from build123d import *

# Parameters (mm, degrees)
SKETCH_1_R          = 6.15
EXTRUDE_1_DEPTH     = 0.2
SKETCH_2_R          = 2.8
EXTRUDE_2_DEPTH     = 0.9
SKETCH_3_R          = 6.15
EXTRUDE_3_DEPTH     = 1.1
EXTRUDE_START       = -0.6
SKETCH_4_R          = 6.15
EXTRUDE_4_DEPTH     = 0.6
CUT_EXTRUDE_START   = -0.2
SKETCH_6_R          = 3.55
SKETCH_6_R_2        = 2.8
CUT_EXTRUDE_2_DEPTH = 0.2
EXTRUDE_START_2     = 7
SKETCH_7_R          = 6.15
SKETCH_7_R_2        = 4.75
EXTRUDE_5_DEPTH     = 7
CHAMFER_4_SIZE      = 2.5
CHAMFER_5_SIZE      = 0.4
CHAMFER_6_SIZE      = 0.4
CHAMFER_7_SIZE      = 1
CHAMFER_8_SIZE      = 0.3


with BuildPart() as part:
    # Sketch 1 → Extrude 1 (new body)
    with BuildSketch(Plane.XY):
        Circle(SKETCH_1_R)
        with BuildLine():
            Line((-0.6, 5.25), (0, 5.85))
            Line((0, 5.85), (0.6, 5.25))
            Line((0.6, 5.25), (0.6, 1.670516387))
            ThreePointArc((0.6, 1.670516387), (0.8875, 1.537195092), (1.146709629, 1.354873436))
            Line((1.146709629, 1.354873436), (4.24663337, 3.144615242))
            Line((4.24663337, 3.144615242), (5.066248612, 2.925))
            Line((5.066248612, 2.925), (4.84663337, 2.105384758))
            Line((4.84663337, 2.105384758), (1.746709629, 0.315642951))
            ThreePointArc((1.746709629, 0.315642951), (1.76791326, 0.158454108), (1.775, 0))
            ThreePointArc((1.775, 0), (1.76791326, -0.158454108), (1.746709629, -0.315642951))
            Line((1.746709629, -0.315642951), (4.84663337, -2.105384758))
            Line((4.84663337, -2.105384758), (5.066248612, -2.925))
            Line((5.066248612, -2.925), (4.24663337, -3.144615242))
            Line((4.24663337, -3.144615242), (1.146709629, -1.354873436))
            ThreePointArc((1.146709629, -1.354873436), (0.8875, -1.537195092), (0.6, -1.670516387))
            Line((0.6, -1.670516387), (0.6, -5.25))
            Line((0.6, -5.25), (0, -5.85))
            Line((0, -5.85), (-0.6, -5.25))
            Line((-0.6, -5.25), (-0.6, -1.670516387))
            ThreePointArc((-0.6, -1.670516387), (-0.8875, -1.537195092), (-1.146709629, -1.354873436))
            Line((-1.146709629, -1.354873436), (-4.24663337, -3.144615242))
            Line((-4.24663337, -3.144615242), (-5.066248612, -2.925))
            Line((-5.066248612, -2.925), (-4.84663337, -2.105384758))
            Line((-4.84663337, -2.105384758), (-1.746709629, -0.315642951))
            ThreePointArc((-1.746709629, -0.315642951), (-1.775, 0), (-1.746709629, 0.315642951))
            Line((-1.746709629, 0.315642951), (-4.84663337, 2.105384758))
            Line((-4.84663337, 2.105384758), (-5.066248612, 2.925))
            Line((-5.066248612, 2.925), (-4.24663337, 3.144615242))
            Line((-4.24663337, 3.144615242), (-1.146709629, 1.354873436))
            ThreePointArc((-1.146709629, 1.354873436), (-0.8875, 1.537195092), (-0.6, 1.670516387))
            Line((-0.6, 1.670516387), (-0.6, 5.25))
        make_face(mode=Mode.SUBTRACT)
    extrude(amount=EXTRUDE_1_DEPTH)

    # Sketch 3 → Extrude 3 (add)
    with BuildSketch(Plane.XY.offset(0.2)):
        Circle(SKETCH_3_R)
        with BuildLine():
            Line((-4.933776406, -2.430606997), (-5.066248612, -2.925))
            Line((-5.066248612, -2.925), (-4.571855609, -3.057472206))
            ThreePointArc((-4.571855609, -3.057472206), (-2.75, -4.763139721), (-0.361920797, -5.488079203))
            Line((-0.361920797, -5.488079203), (0, -5.85))
            Line((0, -5.85), (0.361920797, -5.488079203))
            ThreePointArc((0.361920797, -5.488079203), (2.75, -4.763139721), (4.571855609, -3.057472206))
            Line((4.571855609, -3.057472206), (5.066248612, -2.925))
            Line((5.066248612, -2.925), (4.933776406, -2.430606997))
            ThreePointArc((4.933776406, -2.430606997), (5.5, 0), (4.933776406, 2.430606997))
            Line((4.933776406, 2.430606997), (5.066248612, 2.925))
            Line((5.066248612, 2.925), (4.571855609, 3.057472206))
            ThreePointArc((4.571855609, 3.057472206), (2.75, 4.763139721), (0.361920797, 5.488079203))
            Line((0.361920797, 5.488079203), (0, 5.85))
            Line((0, 5.85), (-0.361920797, 5.488079203))
            ThreePointArc((-0.361920797, 5.488079203), (-2.75, 4.763139721), (-4.571855609, 3.057472206))
            Line((-4.571855609, 3.057472206), (-5.066248612, 2.925))
            Line((-5.066248612, 2.925), (-4.933776406, 2.430606997))
            ThreePointArc((-4.933776406, 2.430606997), (-5.5, 0), (-4.933776406, -2.430606997))
        make_face(mode=Mode.SUBTRACT)
    extrude(amount=EXTRUDE_3_DEPTH)



with BuildPart() as body_2:
    # Sketch 2 → Extrude 2 (new body)
    with BuildSketch(Plane.XY):
        Circle(SKETCH_2_R)
    extrude(amount=EXTRUDE_2_DEPTH)


with BuildPart() as part_1:
    add(part.part)

    add(body_2.part)  # Extrude 4 merges body 2
    # Sketch 4 → Extrude 4 (add)
    with BuildSketch(Plane.XY.offset(EXTRUDE_START)):
        Circle(SKETCH_4_R)
    extrude(amount=EXTRUDE_4_DEPTH)

    # Sketch 6 → Cut-Extrude 2 (cut)
    with BuildSketch(Plane.XY.offset(0.2).offset(CUT_EXTRUDE_START)):
        Circle(SKETCH_6_R)
        Circle(SKETCH_6_R_2, mode=Mode.SUBTRACT)
    extrude(amount=CUT_EXTRUDE_2_DEPTH, mode=Mode.SUBTRACT)

    # Sketch 7 → Extrude 5 (add)
    with BuildSketch(Plane(origin=(0, 0, -0.6), x_dir=(-1, 0, 0), z_dir=(0, 0, -1)).offset(EXTRUDE_START_2)):
        with Locations(Location((0, 0, 0), (0, 0, 180))):
            Circle(SKETCH_7_R)
        Circle(SKETCH_7_R_2, mode=Mode.SUBTRACT)
    extrude(amount=-EXTRUDE_5_DEPTH)

    # Chamfer 4
    chamfer_4_edges = [part_1.edges().sort_by_distance(p)[0] for p in [
        (4.75, 0, -0.6),
    ]]
    chamfer(chamfer_4_edges, length=CHAMFER_4_SIZE)

    # Chamfer 5
    # the kernel refuses this chamfer: 0.4 mm, written as the material it takes off along each edge
    with BuildSketch(Plane(origin=(0, 0, 1.3), x_dir=(1, 0, 0), z_dir=(0, -1, 0))) as chamfer_5_piece_1:
        Polygon((6.15, -CHAMFER_5_SIZE), (6.15 - CHAMFER_5_SIZE, 0), (6.15, 0), align=None)
    revolve(axis=Axis((0, 0, 1.3), (0, 0, 1)), mode=Mode.SUBTRACT)

    # Chamfer 6
    chamfer_6_edges = [part_1.edges().sort_by_distance(p)[0] for p in [
        (-6.15, 0, -7.6),
    ]]
    chamfer(chamfer_6_edges, length=CHAMFER_6_SIZE)

    # Chamfer 7
    # the kernel refuses this chamfer: 1 mm, written as the material it takes off along each edge
    with BuildSketch(Plane(origin=(0, 0, 0.9), x_dir=(1, 0, 0), z_dir=(0, -1, 0))) as chamfer_7_piece_1_section:
        Polygon((2.8, -CHAMFER_7_SIZE), (2.8 - CHAMFER_7_SIZE, 0), (2.8, 0), align=None)
    chamfer_7_piece_1 = revolve(axis=Axis((0, 0, 0.9), (0, 0, 1)), mode=Mode.PRIVATE)
    chamfer_7_piece_1 = split(chamfer_7_piece_1, bisect_by=Plane(origin=(-2.250209939, 0, 0), z_dir=(0, 0, 1)), keep=Keep.TOP, mode=Mode.PRIVATE)
    add(chamfer_7_piece_1, mode=Mode.SUBTRACT)

    # Chamfer 8
    chamfer_8_edges = [part_1.edges().sort_by_distance(p)[0] for p in [
        (4.75, 0, -7.6),
    ]]
    chamfer(chamfer_8_edges, length=CHAMFER_8_SIZE)


solid = part_1.part
Verification items for the finished model (mm, model axes). A direction names the side the tool comes from. Coordinates: 2 decimals unless noted, no trailing zeros. Order: outer loops, then holes, each group sorted by start corner. A loop starts at its lowest first (then second) coordinate and runs counter-clockwise, first axis right, second up. Notation, with made-up numbers: M -21,70.25 L 7,70.25 A22 cw 7,102.25 Z; hole C 68.25,2.25 d3. An arc over 180 degrees is marked long. Write each question's results on one line, items separated by ' | '.
1) Scan lines: line 1 along Y through (x, z) = (0, -3.95); line 2 along Y through (x, z) = (2.75, -6); line 3 along Z through (x, y) = (-1, 4.5). Record each from-to range of solid material in increasing order. Write a range as [from, to].
Solved:
line 1: y = [-6.15, -4.75], [4.75, 6.15] | line 2: y = [-5.5, -3.87], [3.87, 5.5] | line 3: z = [-2.96, 0.2]
2) Access from +Z, -Z, +X, -X, +Y, -Y to the whole of each face (thin tool, end or side, straight path). Record for faces 1 (the face through (-2.72, 4.78, 0.74)), 2 (the face through (0, 0, -0.6)).
Solved:
face 1: +Z | face 2: -Z
3) Gauge pin test, flat ends, axial feed: pin 1 Ø2 at (x, y) = (0.5, -1) entering from -Z; pin 2 Ø2.5 at (x, y) = (-4, 0.5) entering from +Z; pin 3 Ø5 at (x, y) = (-0.5, -2) entering from +Z. Record the tip position at first contact, or that the pin passes through.
Solved:
pin 1: stops at z = -0.6 | pin 2: stops at z = 0.2 | pin 3: stops at z = 0.9
4) Section check A-A on z = 0.5. Record the cut outline in (x, y) (3 decimals).
Solved:
outline: C 0,0 d12.3; C 0,0 d4.4; hole M -5.066,-2.925 L -4.572,-3.057 A5.5 ccw -0.362,-5.488 L 0,-5.85 L 0.362,-5.488 A5.5 ccw 4.572,-3.057 L 5.066,-2.925 L 4.934,-2.431 A5.5 ccw 4.934,2.431 L 5.066,2.925 L 4.572,3.057 A5.5 ccw 0.362,5.488 L 0,5.85 L -0.362,5.488 A5.5 ccw -4.572,3.057 L -5.066,2.925 L -4.934,2.431 A5.5 ccw -4.934,-2.431 Z
5) Section check B-B on y = 0. Record the cut outline in (x, z).
Solved:
outline: M -6.15,-7.2 L -5.75,-7.6 L -5.05,-7.6 L -4.75,-7.3 L -4.75,-3.1 L -2.25,-0.6 L 2.25,-0.6 L 4.75,-3.1 L 4.75,-7.3 L 5.05,-7.6 L 5.75,-7.6 L 6.15,-7.2 L 6.15,0.9 L 5.75,1.3 L 5.5,1.3 L 5.5,0.2 L 3.55,0.2 L 3.55,0 L 2.7,0 L 1.8,0.9 L -1.8,0.9 L -2.7,0 L -3.55,0 L -3.55,0.2 L -5.5,0.2 L -5.5,1.3 L -5.75,1.3 L -6.15,0.9 Z
6) Section check D-D on z = -6.5. Record the cut outline in (x, y).
Solved:
outline: C 0,0 d12.3; hole C 0,0 d9.5
7) Section check C-C on z = -2. Record the cut outline in (x, y), plus the area to 3 significant figures.
Solved:
outline: C 0,0 d12.3; hole C 0,0 d7.3 | area: 77.0 mm²
